from build123d import *

# Parameters (mm, degrees)
MODEL_R               = 4.350000706
MODEL_R_2             = 4.349999799
MAIN_BODY_DEPTH       = 13.2
SIDE_UP_GRAPHIC_DEPTH = 1
HOLE_1_REACH          = 105.138
HOLE_2_REACH          = 92.65


with BuildPart() as part:
    # Model → Main body (new body)
    with BuildSketch(Plane.XY):
        with BuildLine():
            Line((-32.385278451, 85.015032789), (-17.6641047, 76.515992185))
            add(Edge.make_bspline(
                [(-17.6641047, 76.515992185), (-13.888722486, 74.796310284), (-12.180872386, 69.346040832), (-10.138677855, 62.322648799), (-7.341971962, 57.370319929), (-2.311165044, 51.709551581), (2.051636145, 47.586423037), (1.587639106, 43.172213575)],
                knots=[0, 0, 0, 0, 0.279425433, 0.41981198, 0.560237256, 0.707310001, 1, 1, 1, 1], degree=3))
            Line((1.587639106, 43.172213575), (1.587638631, 26.172213575))
            add(Edge.make_bspline(
                [(1.587638631, 26.172213575), (1.626935513, 22.433749487), (-1.504300665, 17.452795295), (-8.065829548, 14.211603151), (-13.487361838, 13.402379484), (-18.908893689, 14.211603727), (-25.470424367, 17.452793212), (-28.601657646, 22.43375075), (-28.56236242, 26.172213575)],
                knots=[0, 0, 0, 0, 0.249525848, 0.374711548, 0.499999996, 0.625288445, 0.750474147, 1, 1, 1, 1], degree=3))
            Line((-28.56236242, 26.172213575), (-28.56236242, 41.723666211))
            add(Edge.make_bspline(
                [(-33.914159524, 51.083510419), (-29.942183369, 47.173551609), (-28.56236242, 41.723666211)],
                knots=[0, 0, 0, 1, 1, 1], degree=2))
            Line((-33.914159524, 51.083510419), (-47.460258007, 58.904368421))
            add(Edge.make_bspline(
                [(-32.385278451, 85.015032789), (-35.600190369, 86.916553219), (-41.474036655, 86.698356276), (-47.559386008, 82.644557032), (-50.972092804, 78.360730829), (-52.985254476, 73.268128205), (-53.475705817, 65.95976879), (-50.710025567, 60.754293561), (-47.460258007, 58.904368421)],
                knots=[0, 0, 0, 0, 0.249337779, 0.374428166, 0.499621296, 0.624814359, 0.749906039, 1, 1, 1, 1], degree=3))
        make_face()
        with Locations((-13.487362418, 22.922213336)):
            Circle(MODEL_R, mode=Mode.SUBTRACT)
        with Locations((-42.737362401, 73.584699743)):
            Circle(MODEL_R_2, mode=Mode.SUBTRACT)
    extrude(amount=MAIN_BODY_DEPTH)

    # Model_4 → Side up graphic (cut)
    with BuildSketch(Plane.XY):
        Polygon((-17.1586416, 60.773364149), (-15.80864309, 58.435095807), (-23.949281442, 53.735095044), (-22.649282205, 51.483428022), (-29.325818765, 52.247530958), (-26.59928106, 58.325030347), (-25.299281823, 56.073363324), align=None)
        Polygon((-21.049281823, 48.71214964), (-12.9086416, 53.412150465), (-11.508643853, 50.987277051), (-19.649280297, 46.287276288), (-18.399280297, 44.122214338), (-25.075818765, 44.886315366), (-22.34928106, 50.963812848), align=None)
        Polygon((-10.0256307, 49.418623945), (-17.875629174, 63.015223523), (-15.537360894, 64.365221998), (-7.68736242, 50.768622419), align=None)
    extrude(amount=SIDE_UP_GRAPHIC_DEPTH, mode=Mode.SUBTRACT)

    # Schizzo3 → Hole 1 (cut, up to next)
    with BuildSketch(Plane(origin=(1.587637901, -4.4e-08, 0), x_dir=(0, 0, -1), z_dir=(0.9999999999999997, -2.789602577989315e-08, 0)), mode=Mode.PRIVATE) as hole_1_sk1:
        with BuildLine():
            Line((-10.95, 32.497213619), (-10.95, 36.847213619))
            Line((-10.95, 36.847213619), (-8.99780105, 38.181209219))
            ThreePointArc((-8.99780105, 38.181209219), (-2.35, 34.672213619), (-8.99780105, 31.163218019))
            Line((-8.99780105, 31.163218019), (-10.95, 32.497213619))
        make_face()
    hole_1_tool1 = extrude(hole_1_sk1.sketch, amount=-HOLE_1_REACH, mode=Mode.PRIVATE) & part.part
    add(hole_1_tool1.solids().sort_by_distance((1.587639, 34.672214, 6.73262))[0], mode=Mode.SUBTRACT)

    # Schizzo4 → Hole 2 (cut, up to next)
    with BuildSketch(Plane(origin=(28.716097743, 49.739103981, 0), x_dir=(0.8660313397108585, -0.499989718532907, 0), z_dir=(0.49998971853290697, 0.8660313397108584, 0)), mode=Mode.PRIVATE) as hole_2_sk1:
        with BuildLine():
            Line((-64.229093026, -10.95), (-59.879093026, -10.95))
            Line((-59.879093026, -10.95), (-58.545097426, -8.99780105))
            ThreePointArc((-58.545097426, -8.99780105), (-62.054093026, -2.35), (-65.563088627, -8.99780105))
            Line((-65.563088627, -8.99780105), (-64.229093026, -10.95))
        make_face()
    hole_2_tool1 = extrude(hole_2_sk1.sketch, amount=-HOLE_2_REACH, mode=Mode.PRIVATE) & part.part
    add(hole_2_tool1.solids().sort_by_distance((-25.024692, 80.765512, 6.73262))[0], mode=Mode.SUBTRACT)


solid = part.part
Design review of the part built by this model. Coordinates are the model's own, in mm. A direction names the side the tool comes from. Round coordinates to 2 decimals unless told otherwise and drop trailing zeros. Order: outer loops, then holes, each group sorted by start corner. A loop starts at its lowest first (then second) coordinate and runs counter-clockwise, first axis right, second up. Notation, with made-up numbers: M 78,81 L 83,81 A24 cw 83,97 Z; hole C -31,35.25 d6. An arc over 180 degrees is marked long. Answer as CSV lines item,"result". Start each with the question number.
1) For pin 1 Ø5 at (y, z) = (77.5, 5.5) entering from +X; pin 2 Ø6.5 at (y, z) = (32, 5) entering from -X; pin 3 Ø5 at (x, z) = (-5.5, 3) entering from -Y, all flat-tipped, find the tip position at first contact; note any pin that passes through.
2) Add section B-B (y = 29.5). Give the boundary of the cut face in (x, z), then the cut area to 3 significant figures.
3) Wall thickness on line 1 along Y through (x, z) = (-13, 8.75); line 2 along X through (y, z) = (76.5, 8); line 3 along Y through (x, z) = (-21.5, 6.6): over which ranges is each line inside the solid? List them lowest first. Write a range as [from, to].
4) The part is to be moulded in two halves that separate along X. For faces 1 (the face through (-25, 51, 0)), 2 (the face through (-12.22, 52.22, 0.49)), 3 (the face through (-28.562, 30, 7)), say which applies: +X half, -X half, draft (parallel to the pull), parting line (faces both ways), or undercut.
5) Add section A-A (z = 6.6). Give the number of separate pieces and of enclosed holes in the cut face, then the cut area to 3 significant figures.
6) Tool access review of faces 4 (the face through (-30, 66.5, 10)), 5 (the face through (-19.82, 56.12, 0.49)): name each direction out of +Z, -Z, +X, -X, +Y, -Y from which nothing blocks a thin tool from reaching the whole face with its end or side.
Resolved:
1,pin 1,"x = -15.39"
1,pin 2,"x = -28.56"
1,pin 3,"y = 14.53"
2,outline,"M -28.56,0 L 1.59,0 L 1.59,13.2 L -28.56,13.2 Z"
2,area,"398 mm^2"
3,line 1,"[13.68, 18.6], [27.24, 31.01], [38.34, 71.42]"
3,line 2,"[-51.62, -45.97], [-39.51, -32.12], [-22.85, -17.63]"
3,line 3,"[15.58, 30.42], [38.92, 78.37]"
4,face 1,"draft"
4,face 2,"undercut"
4,face 3,"-X half"
5,separate pieces,"3"
5,enclosed holes,"2"
5,area,"1,620 mm^2"
6,face 4,"none"
6,face 5,"-Z"
